Verification items for this drawing (mm, ordinates from the low corner). A direction names the side the tool comes from. Give positions to 0.01 mm unless a question says otherwise; leave off trailing zeros. Order: outer loops, then holes, each group sorted by start corner. A loop starts at its lowest first (then second) coordinate and runs counter-clockwise, first axis right, second up. Notation, with made-up numbers: M 40.5,55 L 60.5,55 A20 ccw 60.5,63 Z; hole C 31,85.25 d8. An arc over 180 degrees is marked long. Answer as a JSON object with one key per item and string values.
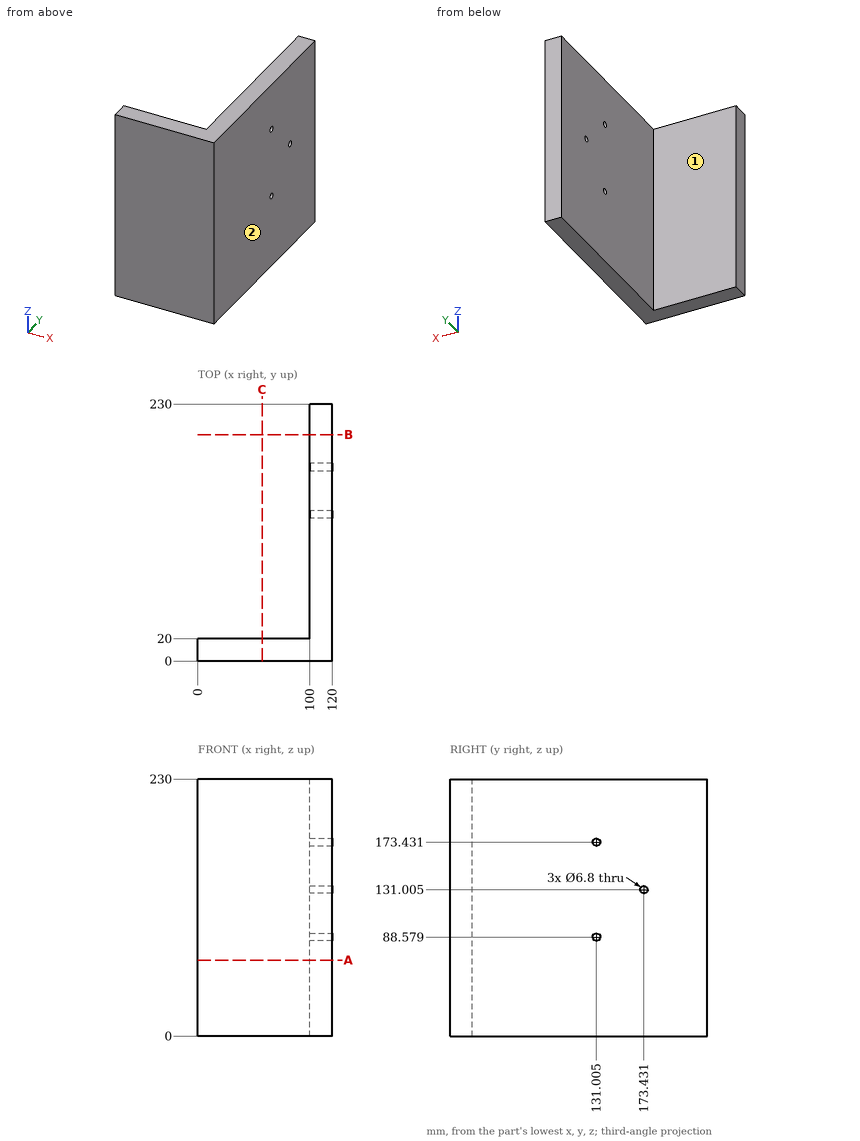
Q1. Section check A-A on z = 68. Record the cut outline in (x, y).
Resolved:
{"outline": "M 0,0 L 120,0 L 120,230 L 100,230 L 100,20 L 0,20 Z"}
Q2. Gauge pin test, flat ends, axial feed: pin 1 Ø3 at (x, z) = (39, 120) entering from +Y; pin 2 Ø5 at (y, z) = (160, 145) entering from -X. Record the tip position at first contact, or that the pin passes through.
Resolved:
{"pin 1": "stops at y = 20", "pin 2": "stops at x = 100"}
Q3. Material ranges on L1, parallel to X at y = 115, z = 71.5; L2, parallel to Y at x = 5, z = 137, recorded low to high.
Resolved:
{"L1": "x = 100 to 120", "L2": "y = 0 to 20"}
Q4. Section check B-B on y = 202.5. Record the cut outline in (x, z).
Resolved:
{"outline": "M 100,0 L 120,0 L 120,230 L 100,230 Z"}
Q5. Section check C-C on x = 57.5. Record the cut outline in (y, z), then the cut area to 3 significant figures.
Resolved:
{"outline": "M 0,0 L 20,0 L 20,230 L 0,230 Z", "area": "4,600 mm²"}
Q6. Tool access check on the marked faces 1 and 2. Record the directions out of +Z, -Z, +X, -X, +Y, -Y that give a thin tool (end or side, any length) a straight path to the whole face; none if there is none.
Resolved:
{"face 1": "+Z, -Z, -X, +Y", "face 2": "+Z, -Z, +X, +Y, -Y"}
